```python
from build123d import *

# Parameters (mm, degrees)
SKETCH2_W           = 25.2
SKETCH2_H           = 15
BOSS_EXTRUDE2_DEPTH = 2
SKETCH3_W           = 2
SKETCH3_H           = 13
BOSS_EXTRUDE3_DEPTH = 7.8
BOSS_EXTRUDE4_DEPTH = 15
SKETCH5_W           = 6.5
SKETCH5_H           = 8.163083502
SKETCH5_W_2         = 2.35
BOSS_EXTRUDE5_DEPTH = 7.8
SKETCH6_W           = 5
SKETCH6_H           = 8.163083502
BOSS_EXTRUDE6_DEPTH = 1.3
SKETCH8_W           = 21.2
SKETCH8_H           = 2
CUT_EXTRUDE1_DEPTH  = 0.5
SKETCH10_R          = 1
CUT_EXTRUDE4_DEPTH  = 6


with BuildPart() as part:
    # Sketch2 → Boss-Extrude2 (new body)
    with BuildSketch(Plane.XY):
        with Locations((-12.6, 7.5)):
            Rectangle(SKETCH2_W, SKETCH2_H)
    extrude(amount=BOSS_EXTRUDE2_DEPTH)

    # Sketch3 → Boss-Extrude3 (add)
    with BuildSketch(Plane.XY.offset(2)):
        Polygon((-25.2, 15), (-25.2, 0), (-23.2, 0), (-23.2, 13), (-23.2, 15), align=None)
        Polygon((-23.2, 15), (-23.2, 13), (-2, 13), (0, 13), (0, 15), align=None)
        with Locations((-1, 6.5)):
            Rectangle(SKETCH3_W, SKETCH3_H)
    extrude(amount=BOSS_EXTRUDE3_DEPTH)

    # Sketch4 → Boss-Extrude4 (add, through all)
    with BuildSketch(Plane(origin=(0, 15, 0), x_dir=(1, 0, 0), z_dir=(0, 1, 0))):
        Polygon((0, 0), (-12.693339498, 12.599654271), (-25.2, 0), align=None)
    extrude(amount=-BOSS_EXTRUDE4_DEPTH)

    # Sketch5 → Boss-Extrude5 (add)
    with BuildSketch(Plane.XY.offset(2)):
        with Locations((-12.6, 4.081541751)):
            Rectangle(SKETCH5_W, SKETCH5_H)
        with Locations((-3.175, 4.081541751)):
            Rectangle(SKETCH5_W_2, SKETCH5_H)
        with Locations((-22.025, 4.081541751)):
            Rectangle(SKETCH5_W_2, SKETCH5_H)
    extrude(amount=BOSS_EXTRUDE5_DEPTH)

    # Sketch6 → Boss-Extrude6 (add)
    with BuildSketch(Plane.XY.offset(2)):
        with Locations((-18.35, 4.081541751)):
            Rectangle(SKETCH6_W, SKETCH6_H)
        with Locations((-6.85, 4.081541751)):
            Rectangle(SKETCH6_W, SKETCH6_H)
    extrude(amount=BOSS_EXTRUDE6_DEPTH)

    # Sketch8 → Cut-Extrude1 (cut)
    with BuildSketch(Plane(origin=(0, 15, 0), x_dir=(1, 0, 0), z_dir=(0, 1, 0))):
        Polygon((-12.682863078, 9.771246548), (-23.2, -0.824090961), (-23.2, -7.8), (-2, -7.8), (-2, -0.832769946), align=None)
        with Locations((-12.6, -8.8)):
            Rectangle(SKETCH8_W, SKETCH8_H)
    extrude(amount=-CUT_EXTRUDE1_DEPTH, mode=Mode.SUBTRACT)

    # Sketch10 → Cut-Extrude4 (cut)
    with BuildSketch(Plane.XY.offset(9.8)):
        with Locations((-12.6, 4)):
            Circle(SKETCH10_R)
    extrude(amount=-CUT_EXTRUDE4_DEPTH, mode=Mode.SUBTRACT)


solid = part.part
```
Work out the finished part from the listing and answer in its coordinate system (mm). A direction names the side the tool comes from. Give positions to 0.01 mm unless a question says otherwise; leave off trailing zeros. Write each loop counter-clockwise with the first axis right and the second up, starting at its lowest first coordinate (ties: lowest second). Pieces come first, ordered by that corner, then holes. Notation, with made-up numbers: (86, -1) -> (116, -1) arc R28 cw to (116, 30) -> close; hole circle Ø6 at (27, 86). An arc over 180 degrees is marked (long way). Write item = value, one per line.
Q1. For a pull along Y with two mould halves and no side action, classify faces 1 (the flat face through (-4.35, 4, 7)), 2 (the flat face through (-16.4, 15, -6.4)), 3 (the flat face through (-13, 13, 6)) as pulls with the +Y half, pulls with the -Y half, needs draft (parallel to the pull), parting line crosses it, or undercut.
Computed values:
face_1 = needs draft
face_2 = pulls with the +Y half
face_3 = undercut
Q2. Section B-B on y = 8.5 is taken. Determine the outline of the cut face in (x, z).
Computed values:
outline = (-25.2, 0) -> (-12.69, -12.6) -> (0, 0) -> (0, 9.8) -> (-2, 9.8) -> (-2, 2) -> (-23.2, 2) -> (-23.2, 9.8) -> (-25.2, 9.8) -> close
Q3. Section D-D on z = -1.25 is taken. Determine the outline of the cut face in (x, y).
Computed values:
outline = (-23.96, 0) -> (-1.26, 0) -> (-1.26, 15) -> (-4.1, 15) -> (-4.1, 14.5) -> (-21.14, 14.5) -> (-21.14, 15) -> (-23.96, 15) -> close
Q4. Consider line 1 along Y through (x, z) = (-12.6, 8.35); line 2 along X through (y, z) = (5.5, 4.25); line 3 along X through (y, z) = (4.5, 4.75). Determine where each line is inside the solid, lowest interval first.
Computed values:
line_1 = 0 to 3, 5 to 8.16, 13 to 14.5
line_2 = -25.2 to -20.85, -15.85 to -9.35, -4.35 to 0
line_3 = -25.2 to -20.85, -15.85 to -13.47, -11.73 to -9.35, -4.35 to 0
Q5. A tool of negligible diameter and unlimited length cuts with its end or side. For faces 4 (the flat face through (0, 7, 5)), 5 (the flat face through (-7.27, 14.75, -4.4)), 6 (the flat face through (-6.258, 7.605, -6.212)), 7 (the flat face through (-13, 11, 2)), 8 (the flat face through (-9.35, 4, 7)), from which of +Z, -Z, +X, -X, +Y, -Y can it reach the whole face along a straight path? Write none if from no direction.
Computed values:
face_4 = +Z, -Z, +X, +Y, -Y
face_5 = +Z, +Y
face_6 = -Z, +X, +Y, -Y
face_7 = +Z
face_8 = +Z, -Y
Q6. Flat-ended cylindrical pins translate along their axes: pin 1 Ø4 at (x, z) = (-7, 0) entering from +Y; pin 2 Ø1.5 at (x, y) = (-17, 4.5) entering from +Z; pin 3 Ø8 at (x, y) = (-5, 9) entering from -Z. Find the tip coordinate at first contact, or state that the pin passes through.
Computed values:
pin_1 = 14.5
pin_2 = 3.3
pin_3 = -8.93
Q7. Section C-C on x = -16.75 is taken. Determine the outline of the cut face in (y, z), and give its area (3 significant figures).
Computed values:
outline = (0, -8.51) -> (15, -8.51) -> (15, -5.67) -> (14.5, -5.67) -> (14.5, 9.8) -> (13, 9.8) -> (13, 2) -> (8.16, 2) -> (8.16, 3.3) -> (0, 3.3) -> close
area = 176 mm^2
Q8. Section A-A on z = 6 is taken. Determine the outline of the cut face in (x, y).
Computed values:
outline = (-25.2, 0) -> (-20.85, 0) -> (-20.85, 8.16) -> (-23.2, 8.16) -> (-23.2, 13) -> (-2, 13) -> (-2, 8.16) -> (-4.35, 8.16) -> (-4.35, 0) -> (0, 0) -> (0, 15) -> (-2, 15) -> (-2, 14.5) -> (-23.2, 14.5) -> (-23.2, 15) -> (-25.2, 15) -> close; (-15.85, 0) -> (-9.35, 0) -> (-9.35, 8.16) -> (-15.85, 8.16) -> close; hole circle Ø2 at (-12.6, 4)
